The listing builds one solid part. Answer for the finished solid, in the listing's coordinates (mm). A direction names the side the tool comes from. Coordinates: 2 decimals unless noted, no trailing zeros. Write each loop counter-clockwise with the first axis right and the second up, starting at its lowest first coordinate (ties: lowest second). Pieces come first, ordered by that corner, then holes.
from build123d import *

# Parameters (mm, degrees)
SWEEP1_PROFILE_R         = 7
BOSS_EXTRUDE1_DEPTH      = 10
BOSS_EXTRUDE1_DEPTH_BACK = 10
SKETCH8_R                = 5


with BuildPart() as part:
    # Sweep1: sweep along a path in Sketch1
    with BuildLine(Plane(origin=(0, 0, 0), x_dir=(1, 0, 0), z_dir=(0, 1, 0))) as sweep1_path:
        Line((0, 0), (-120, 0))
        ThreePointArc((-120, 0), (-141.213203436, 8.786796564), (-150, 30))
        Line((-150, 30), (-150, 80))
    # Sweep1 profile (on start of the path) → Sweep1 (sweep)
    with BuildSketch(Plane(origin=(0, 0, 0), x_dir=(0, 0, -1), z_dir=(-1, 0, 0))):
        Circle(SWEEP1_PROFILE_R)
    sweep(path=sweep1_path.line)

    # Sketch8 → Boss-Extrude1 (add, two sides: drawn at the far end of the back side and taken through both)
    with BuildSketch(Plane(origin=(0, 0, 0), x_dir=(1, 0, 0), z_dir=(0, 1, 0)).offset(-BOSS_EXTRUDE1_DEPTH_BACK)):
        with Locations(Location((-20, 0, 0), (0, 0, 270))):
            Circle(SKETCH8_R)
    extrude(amount=BOSS_EXTRUDE1_DEPTH + BOSS_EXTRUDE1_DEPTH_BACK)


solid = part.part
Q1. Which of the six approach directions +Z, -Z, +X, -X, +Y, -Y give full straight-line access (tool end or side, diameter ignored) to faces 1 (the face through (-143.323, -2.103, -55.35)), 2 (the face through (-61, 0, 7)), 3 (the face through (-18.5, 7.98, 4.77)), 4 (the face through (-24.88, -8.05, -1.08))?
Answers below:
face 1: -Z
face 2: none
face 3: +Y
face 4: -Y
Q2. The part is cut by section D-D, the plane x = -94. Write down the section's boundary in (y, z).
Answers below:
outline: circle Ø14 at (0, 0)
Q3. The part is cut by section A-A, the plane x = -20. Write down the section's boundary in (y, z), then the cut area to 3 significant figures.
Answers below:
outline: (-10, -5) - (-4.9, -5) arc R7 ccw to (4.9, -5) - (10, -5) - (10, 5) - (4.9, 5) arc R7 ccw to (-4.9, 5) - (-10, 5) - close
area: 227 mm2
Q4. The part is cut by section B-B, the plane y = 0. Write down the section's boundary in (x, z), then the cut area to 3 significant figures.
Answers below:
outline: (-157, -80) - (-143, -80) - (-143, -30) arc R23 cw to (-120, -7) - (0, -7) - (0, 7) - (-120, 7) arc R37 ccw to (-157, -30) - close
area: 3,040 mm2
Q5. Given pin 1 (8 mm diameter, centred on x = -94.5, y = -4.5, fed in from -Z); pin 2 (6 mm diameter, centred on x = -137, y = 4.5, fed in from -Z); pin 3 (3 mm diameter, centred on y = -0.5, z = -67, fed in from +X), each flat-ended and moving along its own axis, determine where each tip first touches the part or whether it passes through.
Answers below:
pin 1: stops at z = -6.98
pin 2: stops at z = -16.72
pin 3: stops at x = -143
Q6. The part is cut by section C-C, the plane z = -56.5. Write down the section's boundary in (x, y), then the cut area to 3 significant figures.
Answers below:
outline: circle Ø14 at (-150, 0)
area: 154 mm2
Q7. Find the intervals of material crossed by probe 1 along Z at (x, y) = (-35, 0.5); probe 2 along Z at (x, y) = (-137.5, 5.25); probe 3 along X at (y, z) = (1, -57), in increasing order.
Answers below:
probe 1: z = -6.98 to 6.98
probe 2: z = -11.63 to -0.12
probe 3: x = -156.93 to -143.07
